```python
from build123d import *

# Parameters (mm, degrees)
BOSS_EXTRUDE1_DEPTH      = 2.9
SKETCH1_3_R              = 7
SKETCH1_3_R_2            = 5.5
BOSS_EXTRUDE2_DEPTH      = 10
SKETCH7_R                = 5.5
CUT_EXTRUDE10_DEPTH      = 9
SKETCH8_R                = 6
SKETCH8_R_2              = 5.5
CUT_EXTRUDE11_DEPTH      = 1.8
CUT_EXTRUDE12_DEPTH      = 27.674619931
CUT_EXTRUDE12_DEPTH_BACK = 27.674619931
SKETCH9_W                = 7
SKETCH9_H                = 1.8
CUT_EXTRUDE13_DEPTH      = 27.674619931
CUT_EXTRUDE13_DEPTH_BACK = 27.674619931
CUT_EXTRUDE14_DEPTH      = 10


with BuildPart() as part:
    # Sketch1 → Boss-Extrude1 (new body)
    with BuildSketch(Plane(origin=(0, 0, 0), x_dir=(1, 0, 0), z_dir=(0, 1, 0))):
        with BuildLine():
            Line((-17.959269152, 12), (-11.086554257, -4.59220151))
            ThreePointArc((-11.086554257, -4.59220151), (1.96e-07, -12), (11.086554407, -4.592201147))
            Line((11.086554407, -4.592201147), (17.959269152, 12))
            Line((17.959269152, 12), (17.959269152, 12.01))
            ThreePointArc((17.959269152, 12.01), (17.619614776, 14.59281423), (16.623747761, 17))
            Line((16.623747761, 17), (-16.623747761, 17))
            ThreePointArc((-16.623747761, 17), (-17.619614776, 14.59281423), (-17.959269152, 12.01))
            Line((-17.959269152, 12.01), (-17.959269152, 12))
        make_face()
    extrude(amount=BOSS_EXTRUDE1_DEPTH)

    # Sketch1_3 → Boss-Extrude2 (add)
    with BuildSketch(Plane(origin=(0, 0, 0), x_dir=(1, 0, 0), z_dir=(0, 1, 0))):
        with Locations(Location((0, 0, 0), (0, 0, 270))):
            Circle(SKETCH1_3_R)
        Circle(SKETCH1_3_R_2)
    extrude(amount=BOSS_EXTRUDE2_DEPTH)

    # Sketch7 → Cut-Extrude10 (cut)
    with BuildSketch(Plane(origin=(0, 10, 0), x_dir=(1, 0, 0), z_dir=(0, 1, 0))):
        with Locations(Location((0, 0, 0), (0, 0, 270))):
            Circle(SKETCH7_R)
    extrude(amount=-CUT_EXTRUDE10_DEPTH, mode=Mode.SUBTRACT)

    # Sketch8 → Cut-Extrude11 (cut)
    with BuildSketch(Plane(origin=(0, 9, 0), x_dir=(1, 0, 0), z_dir=(0, 1, 0))):
        with Locations(Location((0, 0, 0), (0, 0, 270))):
            Circle(SKETCH8_R)
        with Locations(Location((0, 0, 0), (0, 0, 270))):
            Circle(SKETCH8_R_2, mode=Mode.SUBTRACT)
    extrude(amount=-CUT_EXTRUDE11_DEPTH, mode=Mode.SUBTRACT)

    # Sketch9 → Cut-Extrude12 (cut, two sides: drawn at the far end of the back side and taken through both)
    with BuildSketch(Plane.XY.offset(-CUT_EXTRUDE12_DEPTH_BACK)):
        with Locations((0, 8.1)):
            Rectangle(SKETCH9_W, SKETCH9_H)
    extrude(amount=CUT_EXTRUDE12_DEPTH + CUT_EXTRUDE12_DEPTH_BACK, mode=Mode.SUBTRACT)

    # Sketch10 → Cut-Extrude13 (cut, two sides: drawn at the far end of the back side and taken through both)
    with BuildSketch(Plane(origin=(0, 0, 0), x_dir=(0, 0, -1), z_dir=(1, 0, 0)).offset(-CUT_EXTRUDE13_DEPTH_BACK)):
        Polygon((17, 0), (7, 2.9), (17, 2.9), align=None)
    extrude(amount=CUT_EXTRUDE13_DEPTH + CUT_EXTRUDE13_DEPTH_BACK, mode=Mode.SUBTRACT)

    # Sketch11 → Cut-Extrude14 (cut)
    with BuildSketch(Plane(origin=(0, 0, 0), x_dir=(0, 0, -1), z_dir=(1, 0, 0))):
        Polygon((-2.1, 10.6), (2.1, 10.6), (2.1, 9.8), (1.428720295, 9), (-1.428720295, 9), (-2.1, 9.8), align=None)
    extrude(amount=CUT_EXTRUDE14_DEPTH, mode=Mode.SUBTRACT)


solid = part.part
```
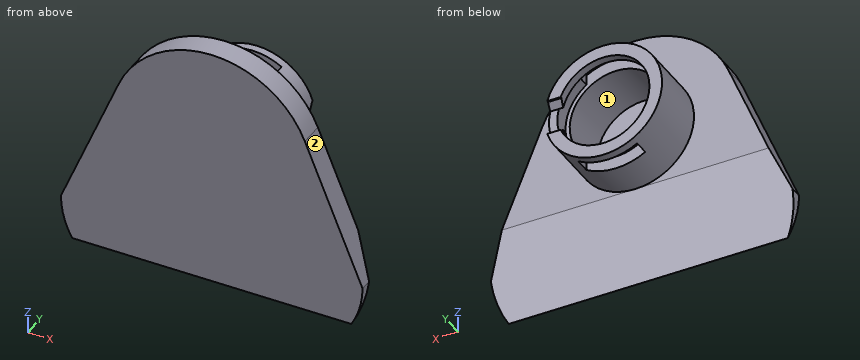
CAD build for the part. Positions are in the model's coordinates, mm. Face numbers are marked on the shaded views. A direction names the side the tool comes from. Give positions to 0.01 mm unless a question says otherwise; leave off trailing zeros. Loops run counter-clockwise (first coordinate to the right, second up) from the corner with the lowest first, then second, coordinate; pieces in that order, holes last. Notation, with made-up numbers: M -4,17 L 13,17 A17 cw 13,42 Z; hole C 17,-2 d7. An arc over 180 degrees is marked long. Use one line per item in the form item = value.
Item 1: Slice it at B-B (z = -4). List the corners of the cut face in (x, y).
Determined:
outline = M -14.65,0 L 14.65,0 L 14.65,2.9 L 5.74,2.9 L 5.74,10 L 3.77,10 L 3.77,9 L 4.47,9 L 4.47,7.2 L 3.77,7.2 L 3.77,1 L -3.77,1 L -3.77,7.2 L -4.47,7.2 L -4.47,9 L -3.77,9 L -3.77,10 L -5.74,10 L -5.74,2.9 L -14.65,2.9 Z
Item 2: Slice it at A-A (y = 2.5). List the corners of the cut face in (x, z).
Determined:
outline = M -16.46,-8.38 L 16.46,-8.38 L 11.09,4.59 A12 ccw -11.09,4.59 Z; hole C 0,0 d11
Item 3: Slice it at D-D (z = 0). List the corners of the cut face in (x, y).
Determined:
outline = M -12.99,0 L 12.99,0 L 12.99,2.9 L 7,2.9 L 7,9 L 6,9 L 6,7.2 L 5.5,7.2 L 5.5,1 L -5.5,1 L -5.5,7.2 L -6,7.2 L -6,9 L -5.5,9 L -5.5,10 L -7,10 L -7,2.9 L -12.99,2.9 Z
Item 4: Drill centre lines: probe 1 along Z at (x, y) = (0, 9.45); probe 2 along Y at (x, z) = (-6, -3.75). Where is each one in solid material? Low to high. Write a range as from..to.
Determined:
probe_1 = -7..-5.5, 5.5..7
probe_2 = 0..2.9
Item 5: Which spindle directions (+Z, -Z, +X, -X, +Y, -Y) get a long thin tool onto all of the face, cutting with end or side? Do the marked faces 1 and 2. Say none if no direction does.
Determined:
face_1 = +Y
face_2 = +Z, +X, +Y, -Y
Item 6: Flat gauge pins, fed straight in: pin 1 (5 mm diameter, centred on y = 2.5, z = -6, fed in from -X); pin 2 (1.5 mm diameter, centred on x = -7, y = 6.5, fed in from +Z); pin 3 (1 mm diameter, centred on y = 7.5, z = -5, fed in from +X). Where does each tip first touch, or does it go through?
Determined:
pin_1 = -16.51
pin_2 = 3.15
pin_3 = 5.36
Item 7: Slice it at C-C (x = -4). List the corners of the cut face in (y, z), plus the area to 3 significant figures.
Determined:
outline = M 0,-17 L 2.9,-7 L 2.9,-5.74 L 10,-5.74 L 10,-3.77 L 9,-3.77 L 9,-4.47 L 7.2,-4.47 L 7.2,-3.77 L 1,-3.77 L 1,3.77 L 7.2,3.77 L 7.2,4.47 L 9,4.47 L 9,3.77 L 10,3.77 L 10,5.74 L 2.9,5.74 L 2.9,11.31 L 0,11.31 Z
area = 78.7 mm2
